Job drawing, mm, ordinate dimensions from the low corner. One solid piece. A direction names the side the tool comes from. Coordinates: 2 decimals unless noted, no trailing zeros. Loops run counter-clockwise (first coordinate to the right, second up) from the corner with the lowest first, then second, coordinate; pieces in that order, holes last. Notation, with made-up numbers: (-11.75, 46.25) - (4.25, 46.25) arc R14 cw to (4.25, 55.25) - close; hole circle Ø11 at (12.5, 33). An arc over 180 degrees is marked (long way). Use a Markdown table: item, result. Add a question column.
1) Band-saw the part on A-A (y = 43.5). Give the cut face in (x, z).
2) Band-saw the part on D-D (z = 15.75). Give the cut face in (x, y).
3) Band-saw the part on B-B (z = 1.75). Give the cut face in (x, y), plus the area to 3 significant figures.
4) Pull direction Y, two halves, no side cores. Call the marked faces 3, 4 and 5: +Y half, -Y half, draft (parallel to the pull), parting line (faces both ways), or undercut.
5) Drop flat-ended pins along their axis: P1, Ø8, axis at x = 53.75, y = 3.75, coming from the +Z side; P2, Ø4, axis at x = 53.5, y = 4.5, coming from the -Z side; P3, Ø4, axis at y = 41.5, z = 2.5, coming from the -X side; P4, Ø1, axis at y = 28, z = 1, coming from the -X side. Give the stop position or say it passes through.
6) Probe probe 1 along Y at (x, z) = (3.75, 8.5); probe 2 along X at (y, z) = (45, 2.25); probe 3 along Z at (x, y) = (31, 19). List the from-to ranges inside material, lowest first. Write a range as [from, to].
7) Tool access for the marked faces 1 and 2: list every direction of +Z, -Z, +X, -X, +Y, -Y with a clear straight run to the whole face (end or side of a thin tool).
8) Band-saw the part on C-C (x = 25). Give the cut face in (y, z).
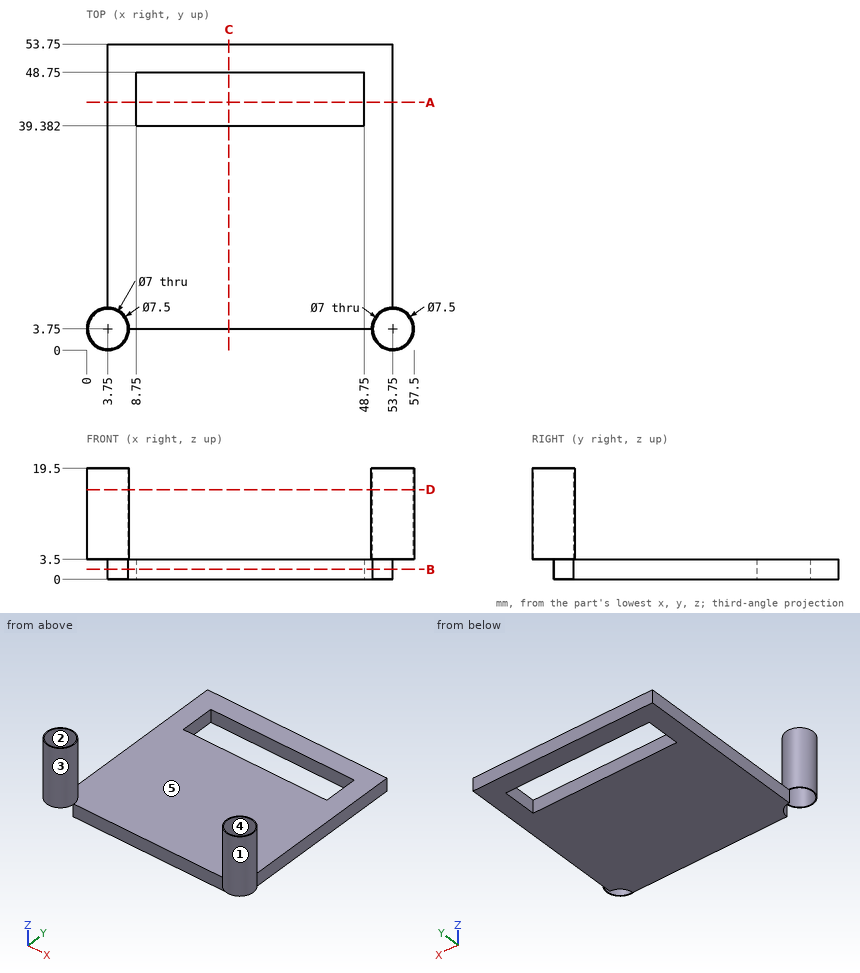
Answer block:
| question | item | result |
|---|---|---|
| 1 | outline | (3.75, 0) - (8.75, 0) - (8.75, 3.5) - (3.75, 3.5) - close; (48.75, 0) - (53.75, 0) - (53.75, 3.5) - (48.75, 3.5) - close |
| 2 | outline | circle Ø7.5 at (3.75, 3.75); circle Ø7.5 at (53.75, 3.75); hole circle Ø7 at (3.75, 3.75); hole circle Ø7 at (53.75, 3.75) |
| 3 | outline | (3.75, 7.25) arc R3.5 cw to (7.25, 3.75) - (50.25, 3.75) arc R3.5 cw to (53.75, 7.25) - (53.75, 53.75) - (3.75, 53.75) - close; hole (8.75, 39.38) - (48.75, 39.38) - (48.75, 48.75) - (8.75, 48.75) - close |
| 3 | area | 2,110 mm2 |
| 4 | face 3 | parting line |
| 4 | face 4 | undercut |
| 4 | face 5 | draft |
| 5 | P1 | z = 19.5 |
| 5 | P2 | through |
| 5 | P3 | x = 3.75 |
| 5 | P4 | x = 3.75 |
| 6 | probe 1 | [0, 0.25], [7.25, 7.5] |
| 6 | probe 2 | [3.75, 8.75], [48.75, 53.75] |
| 6 | probe 3 | [0, 3.5] |
| 7 | face 1 | +Z |
| 7 | face 2 | +Z, -Z |
| 8 | outline | (3.75, 0) - (39.38, 0) - (39.38, 3.5) - (3.75, 3.5) - close; (48.75, 0) - (53.75, 0) - (53.75, 3.5) - (48.75, 3.5) - close |
